```python
from build123d import *

# Parameters (mm, degrees)
BOSS_EXTRUDE1_DEPTH      = 10
BOSS_EXTRUDE1_DEPTH_BACK = 10
SKETCH1_R                = 6
SKETCH2_R                = 3
CUT_EXTRUDE1_DEPTH       = 10
SKETCH3_R                = 2
CUT_EXTRUDE2_DEPTH       = 10
CUT_EXTRUDE4_REACH       = 15.115
CUT_EXTRUDE4_END_RADIUS  = 6
SKETCH4_R                = 1
FILLET1_R                = 0.5
SKETCH5_R                = 2.1
CUT_EXTRUDE7_DEPTH       = 2


with BuildPart() as part:
    # Sketch1 → Boss-Extrude1 (new, two sides: drawn at the far end of the back side and taken through both)
    with BuildSketch(Plane(origin=(0, 0, 0), x_dir=(0, 0, -1), z_dir=(1, 0, 0)).offset(-BOSS_EXTRUDE1_DEPTH_BACK)):
        Circle(SKETCH1_R)
    extrude(amount=BOSS_EXTRUDE1_DEPTH + BOSS_EXTRUDE1_DEPTH_BACK)

    # Sketch2 → Cut-Extrude1 (cut)
    with BuildSketch(Plane(origin=(10, 0, 0), x_dir=(0, 0, -1), z_dir=(1, 0, 0))):
        Circle(SKETCH2_R)
    extrude(amount=-CUT_EXTRUDE1_DEPTH, mode=Mode.SUBTRACT)

    # Sketch3 → Cut-Extrude2 (cut)
    with BuildSketch(Plane.ZY.offset(10)):
        Circle(SKETCH3_R)
    extrude(amount=-CUT_EXTRUDE2_DEPTH, mode=Mode.SUBTRACT)

    # Cut-Extrude4: up to this cylinder (the profile starts inside it)
    cut_extrude4_end = Plane(origin=(0, 0, 0), z_dir=(1, 0, 0)) * Cylinder(CUT_EXTRUDE4_END_RADIUS, 55.23, mode=Mode.PRIVATE)
    # Sketch4 → Cut-Extrude4 (cut, up to the surface)
    with BuildSketch(Plane(origin=(0, 0, 0), x_dir=(1, 0, 0), z_dir=(0, 1, 0)), mode=Mode.PRIVATE) as cut_extrude4_sk1:
        with Locations(Location((-6, 0, 0), (0, 0, 90))):
            Circle(SKETCH4_R)
    cut_extrude4_tool1 = extrude(cut_extrude4_sk1.sketch, amount=CUT_EXTRUDE4_REACH, mode=Mode.PRIVATE) & cut_extrude4_end
    add(cut_extrude4_tool1.solids().sort_by_distance((-6, 0, 0))[0], mode=Mode.SUBTRACT)
    # Sketch4 → Cut-Extrude4 (cut, up to the surface)
    with BuildSketch(Plane(origin=(0, 0, 0), x_dir=(1, 0, 0), z_dir=(0, 1, 0)), mode=Mode.PRIVATE) as cut_extrude4_sk2:
        with Locations(Location((6, 0, 0), (0, 0, 90))):
            Circle(SKETCH4_R)
    cut_extrude4_tool2 = extrude(cut_extrude4_sk2.sketch, amount=CUT_EXTRUDE4_REACH, mode=Mode.PRIVATE) & cut_extrude4_end
    add(cut_extrude4_tool2.solids().sort_by_distance((6, 0, 0))[0], mode=Mode.SUBTRACT)

    # Fillet1
    fillet1_edges = [part.edges().sort_by_distance(p)[0] for p in [
        (-10, 0, -2),
        (-10, 0, 6),
        (10, 0, 6),
        (10, 0, 3),
    ]]
    fillet(fillet1_edges, radius=FILLET1_R)

    # Sketch5 → Cut-Extrude7 (cut)
    with BuildSketch(Plane(origin=(0, 6, 0), x_dir=(1, 0, 0), z_dir=(0, 1, 0))):
        with Locations(Location((-6, 0, 0), (0, 0, 270))):
            Circle(SKETCH5_R)
        with Locations(Location((6, 0, 0), (0, 0, 270))):
            Circle(SKETCH5_R)
    extrude(amount=-CUT_EXTRUDE7_DEPTH, mode=Mode.SUBTRACT)


solid = part.part
```
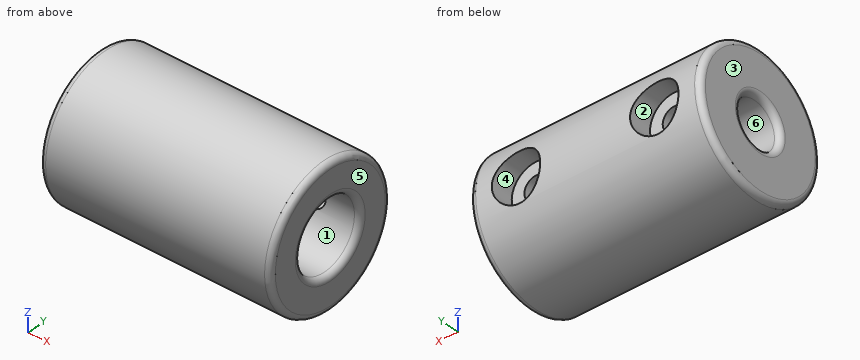
Geometry: final body of the model. Coordinates: model frame, mm. Face numbers are marked on the shaded views. A direction names the side the tool comes from. Round coordinates to 2 decimals unless told otherwise and drop trailing zeros. Write each loop counter-clockwise with the first axis right and the second up, starting at its lowest first coordinate (ties: lowest second). Pieces come first, ordered by that corner, then holes. Notation, with made-up numbers: M 32.5,26.5 L 53.5,26.5 A21 ccw 53.5,60.5 Z; hole C 29.25,11.5 d5. An arc over 180 degrees is marked long. Answer in a Markdown table with one row per item. Add a question column.
(1) Cut plane A-A, the plane y = 0. Return the cut outline in (x, z), then the cut area to 3 significant figures.
(2) Contact query for flat-ended pins moving along their axis: pin 1 (1.6 mm diameter, centred on x = 6, z = 0, fed in from +Y); pin 2 (2.5 mm diameter, centred on y = 0, z = 0, fed in from +X); pin 3 (1.5 mm diameter, centred on x = 6.5, y = -1, fed in from -Z); pin 4 (2 mm diameter, centred on x = -5.5, z = -0.5, fed in from +Y). Output: stop coordinate, or through.
(3) Ray query, L1, parallel to X at y = 3.7, z = 0; L2, parallel to X at y = 5.15, z = 0; L3, parallel to X at y = -2.75, z = -1. Return the intervals inside material, ascending.
(4) Reachability of the marked faces 1, 2 and 3 from +Z, -Z, +X, -X, +Y, -Y: full face, straight path, thin tool, end or side. Return the list, or none.
(5) Cut plane C-C, the plane z = 0. Give the number of separate pieces and of enclosed holes in the cut face, then the cut area to 3 significant figures.
(6) Cut plane D-D, the plane x = 6. Return the cut outline in (y, z).
(7) Draft query along X for the marked faces 4, 5 and 6. Return one class per face: pulls with the +X half, pulls with the -X half, needs draft (parallel to the pull), parting line crosses it, or undercut.
(8) Cut plane B-B, the plane x = 1.25. Return the cut outline in (y, z).
Established:
| question | item | result |
|---|---|---|
| 1 | outline | M -10,-5.5 A0.5 ccw -9.5,-6 L 9.5,-6 A0.5 ccw 10,-5.5 L 10,-3.5 A0.5 ccw 9.5,-3 L 0,-3 L 0,-2 L -9.5,-2 A0.5 ccw -10,-2.5 Z; M -10,2.5 A0.5 ccw -9.5,2 L 0,2 L 0,3 L 9.5,3 A0.5 ccw 10,3.5 L 10,5.5 A0.5 ccw 9.5,6 L -9.5,6 A0.5 ccw -10,5.5 Z |
| 1 | area | 140 mm² |
| 2 | pin 1 | y = -2.89 |
| 2 | pin 2 | through |
| 2 | pin 3 | z = -5.99 |
| 2 | pin 4 | y = 4 |
| 3 | L1 | -10 to -7, -5 to 5, 7 to 10 |
| 3 | L2 | -10 to -8.1, -3.9 to 3.9, 8.1 to 10 |
| 3 | L3 | -10 to 0 |
| 4 | face 1 | +X |
| 4 | face 2 | +Y |
| 4 | face 3 | +Z, -Z, -X, +Y, -Y |
| 5 | separate pieces | 4 |
| 5 | enclosed holes | 0 |
| 5 | area | 117 mm² |
| 6 | outline | M 2.83,-1 A3 cw long 2.83,1 L 4,1 L 4,2.1 L 5.62,2.1 A6 ccw long 5.62,-2.1 L 4,-2.1 L 4,-1 Z |
| 7 | face 4 | undercut |
| 7 | face 5 | pulls with the +X half |
| 7 | face 6 | needs draft |
| 8 | outline | C 0,0 d12; hole C 0,0 d6 |
